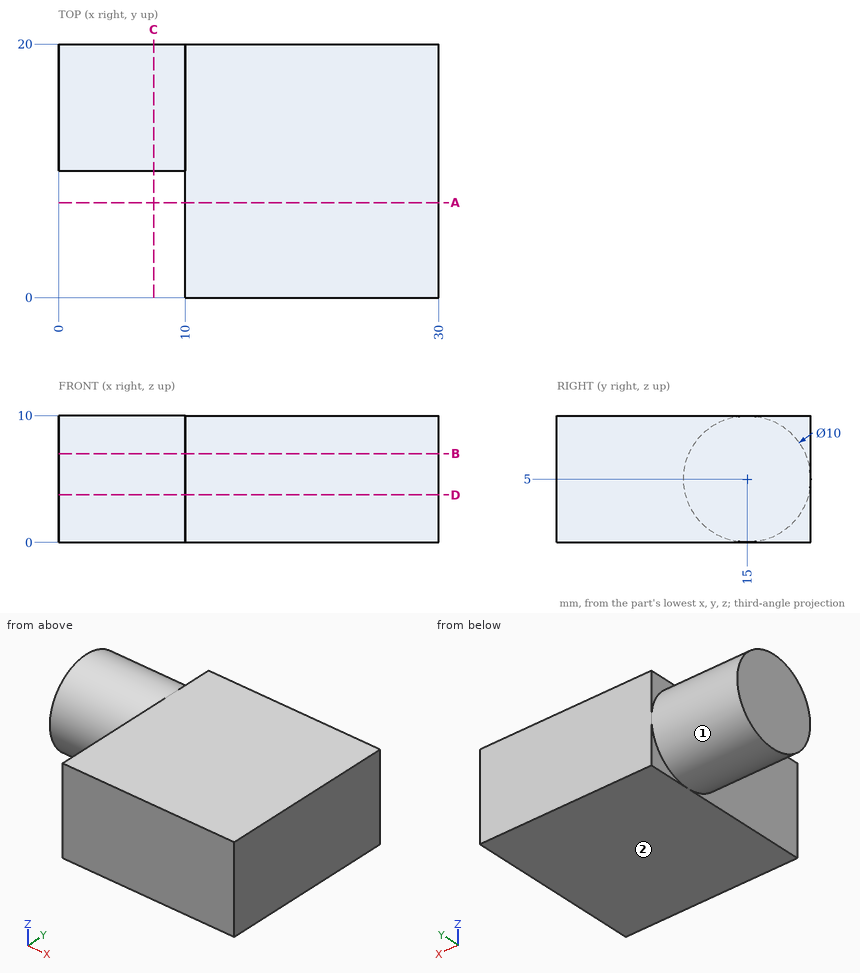
Job drawing, mm, ordinate dimensions from the low corner. One solid piece. A direction names the side the tool comes from. Round coordinates to 2 decimals unless told otherwise and drop trailing zeros. Loops run counter-clockwise (first coordinate to the right, second up) from the corner with the lowest first, then second, coordinate; pieces in that order, holes last. Notation, with made-up numbers: (-31.75, 45.25) -> (-21.75, 45.25) arc R10 cw to (-21.75, 59.25) -> close; hole circle Ø8 at (42, 62). An arc over 180 degrees is marked (long way). Use a Markdown table: item, result.
1) Cut at A-A, the plane y = 7.5. List the corners of the cut face in (x, z), and give its area (3 significant figures).
The answers:
| item | result |
|---|---|
| outline | (10, 0) -> (30, 0) -> (30, 10) -> (10, 10) -> close |
| area | 200 mm2 |
2) Tool access for the marked faces 1 and 2: list every direction of +Z, -Z, +X, -X, +Y, -Y with a clear straight run to the whole face (end or side of a thin tool).
The answers:
| item | result |
|---|---|
| face 1 | -X |
| face 2 | -Z, +X, -X, +Y, -Y |
3) Cut at D-D, the plane z = 3.75. List the corners of the cut face in (x, y).
The answers:
| item | result |
|---|---|
| outline | (0, 10.16) -> (10, 10.16) -> (10, 0) -> (30, 0) -> (30, 20) -> (10, 20) -> (10, 19.84) -> (0, 19.84) -> close |
4) Cut at B-B, the plane z = 7. List the corners of the cut face in (x, y), and give its area (3 significant figures).
The answers:
| item | result |
|---|---|
| outline | (0, 10.42) -> (10, 10.42) -> (10, 0) -> (30, 0) -> (30, 20) -> (10, 20) -> (10, 19.58) -> (0, 19.58) -> close |
| area | 492 mm2 |
5) Drop flat-ended pins along their axis: pin 1 Ø5 at (x, z) = (18, 1.5) entering from -Y; pin 2 Ø3 at (y, z) = (6.5, 6) entering from -X. Give the stop position or say it passes through.
The answers:
| item | result |
|---|---|
| pin 1 | stops at y = 0 |
| pin 2 | stops at x = 10 |
6) Probe line 1 (X direction, y = 3, z = 2); line 2 (Y direction, x = 2, z = 4); line 3 (Y direction, x = 4.75, z = 8.5). List the from-to ranges inside material, lowest first. Write a range as [from, to].
The answers:
| item | result |
|---|---|
| line 1 | x = [10, 30] |
| line 2 | y = [10.1, 19.9] |
| line 3 | y = [11.43, 18.57] |
7) Cut at C-C, the plane x = 7.5. List the corners of the cut face in (y, z), and give its area (3 significant figures).
The answers:
| item | result |
|---|---|
| outline | circle Ø10 at (15, 5) |
| area | 78.5 mm2 |
